Part model, mm, in its own coordinate system. A direction names the side the tool comes from. Round coordinates to 2 decimals unless told otherwise and drop trailing zeros. Order: outer loops, then holes, each group sorted by start corner. A loop starts at its lowest first (then second) coordinate and runs counter-clockwise, first axis right, second up. Notation, with made-up numbers: (30.5, 55) -> (78.5, 55) arc R21 cw to (78.5, 67) -> close; hole circle Ø11 at (6.25, -14). An arc over 180 degrees is marked (long way). Use CSV: the item, a comma, the result in double quotes.
```python
from build123d import *

# Parameters (mm, degrees)
SKETCH1_R              = 2.035533906
SKETCH1_R_2            = 1.5
BOSS_EXTRUDE1_DEPTH    = 1
SKETCH1_3_R            = 1.5
BOSS_EXTRUDE2_DEPTH    = 2
BOSS_EXTRUDE2_2_DEPTH  = 2
BOSS_EXTRUDE2_3_DEPTH  = 2
BOSS_EXTRUDE2_4_DEPTH  = 2
BOSS_EXTRUDE2_5_DEPTH  = 2
BOSS_EXTRUDE2_6_DEPTH  = 2
BOSS_EXTRUDE2_7_DEPTH  = 2
BOSS_EXTRUDE2_8_DEPTH  = 2
BOSS_EXTRUDE2_9_DEPTH  = 2
BOSS_EXTRUDE2_10_DEPTH = 2
BOSS_EXTRUDE2_11_DEPTH = 2
BOSS_EXTRUDE2_12_DEPTH = 2
BOSS_EXTRUDE2_13_DEPTH = 2
BOSS_EXTRUDE2_14_DEPTH = 2
BOSS_EXTRUDE2_15_DEPTH = 2
BOSS_EXTRUDE2_16_DEPTH = 2
SKETCH1_4_W            = 20
SKETCH1_4_H            = 20
BOSS_EXTRUDE3_DEPTH    = 1


with BuildPart() as part:
    # Sketch1 → Boss-Extrude1 (new body)
    with BuildSketch(Plane(origin=(0, 0, 0), x_dir=(1, 0, 0), z_dir=(0, 1, 0))):
        Polygon((1, 7.499999998), (1, 12.5), (1, 17.5), (0, 17.5), (0, 0), (20, 0), (20, 20), (2.5, 20), (2.5, 19), (7.5, 19), (12.500000017, 19), (17.5, 19), (19, 19), (19, 17.5), (19, 12.5), (19, 7.5), (19, 2.5), (19, 1), (17.5, 1), (12.49999999, 1), (7.5, 1), (2.5, 1), (1, 1), (1, 2.5), align=None)
        with Locations((5, 5)):
            Circle(SKETCH1_R)
        with Locations((5, 5)):
            Circle(SKETCH1_R_2, mode=Mode.SUBTRACT)
        with Locations((5, 10)):
            Circle(SKETCH1_R)
        with Locations((5, 10)):
            Circle(SKETCH1_R_2, mode=Mode.SUBTRACT)
        with BuildLine():
            ThreePointArc((3.560660176, 16.439339833), (2.964466094, 15.000000004), (3.560660171, 13.560660172))
            Line((3.560660172, 13.560660172), (3.939339828, 13.939339828))
            ThreePointArc((3.939339828, 13.939339828), (3.939339828, 16.060660172), (6.060660172, 16.060660172))
            Line((6.060660172, 16.060660172), (6.439339828, 16.439339828))
            ThreePointArc((6.439339828, 16.439339829), (5.000000003, 17.035533906), (3.560660176, 16.439339833))
        make_face()
        with BuildLine():
            Line((3.939339828, 13.939339828), (3.560660172, 13.560660172))
            ThreePointArc((3.560660171, 13.560660172), (5, 12.964466094), (6.439339828, 13.560660172))
            ThreePointArc((6.439339828, 13.560660172), (6.880588113, 14.221034898), (7.035533906, 15))
            ThreePointArc((7.035533906, 15), (6.880588113, 15.778965102), (6.439339828, 16.439339829))
            Line((6.439339828, 16.439339828), (6.060660172, 16.060660172))
            ThreePointArc((6.060660172, 16.060660172), (6.385819299, 15.574025149), (6.5, 15))
            ThreePointArc((6.5, 15), (5.574025149, 13.614180701), (3.939339828, 13.939339828))
        make_face()
        with Locations((10, 5)):
            Circle(SKETCH1_R)
        with Locations((10, 5)):
            Circle(SKETCH1_R_2, mode=Mode.SUBTRACT)
        with Locations((15, 5)):
            Circle(SKETCH1_R)
        with Locations((15, 5)):
            Circle(SKETCH1_R_2, mode=Mode.SUBTRACT)
        with Locations((15, 15)):
            Circle(SKETCH1_R)
        with Locations((15, 15)):
            Circle(SKETCH1_R_2, mode=Mode.SUBTRACT)
        with Locations((15, 10)):
            Circle(SKETCH1_R)
        with Locations((15, 10)):
            Circle(SKETCH1_R_2, mode=Mode.SUBTRACT)
        with Locations((10, 10)):
            Circle(SKETCH1_R)
        with Locations((10, 10)):
            Circle(SKETCH1_R_2, mode=Mode.SUBTRACT)
        with Locations((10, 15)):
            Circle(SKETCH1_R)
        with Locations((10, 15)):
            Circle(SKETCH1_R_2, mode=Mode.SUBTRACT)
        Polygon((0, 17.5), (1, 17.5), (1, 19), (2.5, 19), (2.5, 20), (0, 20), align=None)
    extrude(amount=-BOSS_EXTRUDE1_DEPTH)



with BuildPart() as body_2:
    # Sketch1_3 → Boss-Extrude2 (new body)
    with BuildSketch(Plane(origin=(0, 0, 0), x_dir=(1, 0, 0), z_dir=(0, 1, 0))):
        with Locations((2.5, 12.5)):
            Circle(SKETCH1_3_R)
    extrude(amount=BOSS_EXTRUDE2_DEPTH)


with BuildPart() as body_3:
    # Sketch1_3 → Boss-Extrude2 2 (new body)
    with BuildSketch(Plane(origin=(0, 0, 0), x_dir=(1, 0, 0), z_dir=(0, 1, 0))):
        with Locations((2.5, 17.5)):
            Circle(SKETCH1_3_R)
    extrude(amount=BOSS_EXTRUDE2_2_DEPTH)


with BuildPart() as body_4:
    # Sketch1_3 → Boss-Extrude2 3 (new body)
    with BuildSketch(Plane(origin=(0, 0, 0), x_dir=(1, 0, 0), z_dir=(0, 1, 0))):
        with Locations((7.5, 12.5)):
            Circle(SKETCH1_3_R)
    extrude(amount=BOSS_EXTRUDE2_3_DEPTH)


with BuildPart() as body_5:
    # Sketch1_3 → Boss-Extrude2 4 (new body)
    with BuildSketch(Plane(origin=(0, 0, 0), x_dir=(1, 0, 0), z_dir=(0, 1, 0))):
        with Locations((2.5, 7.5)):
            Circle(SKETCH1_3_R)
    extrude(amount=BOSS_EXTRUDE2_4_DEPTH)


with BuildPart() as body_6:
    # Sketch1_3 → Boss-Extrude2 5 (new body)
    with BuildSketch(Plane(origin=(0, 0, 0), x_dir=(1, 0, 0), z_dir=(0, 1, 0))):
        with Locations((7.5, 17.5)):
            Circle(SKETCH1_3_R)
    extrude(amount=BOSS_EXTRUDE2_5_DEPTH)


with BuildPart() as body_7:
    # Sketch1_3 → Boss-Extrude2 6 (new body)
    with BuildSketch(Plane(origin=(0, 0, 0), x_dir=(1, 0, 0), z_dir=(0, 1, 0))):
        with Locations((2.5, 2.5)):
            Circle(SKETCH1_3_R)
    extrude(amount=BOSS_EXTRUDE2_6_DEPTH)


with BuildPart() as body_8:
    # Sketch1_3 → Boss-Extrude2 7 (new body)
    with BuildSketch(Plane(origin=(0, 0, 0), x_dir=(1, 0, 0), z_dir=(0, 1, 0))):
        with Locations((12.5, 12.5)):
            Circle(SKETCH1_3_R)
    extrude(amount=BOSS_EXTRUDE2_7_DEPTH)


with BuildPart() as body_9:
    # Sketch1_3 → Boss-Extrude2 8 (new body)
    with BuildSketch(Plane(origin=(0, 0, 0), x_dir=(1, 0, 0), z_dir=(0, 1, 0))):
        with Locations((7.5, 7.5)):
            Circle(SKETCH1_3_R)
    extrude(amount=BOSS_EXTRUDE2_8_DEPTH)


with BuildPart() as body_10:
    # Sketch1_3 → Boss-Extrude2 9 (new body)
    with BuildSketch(Plane(origin=(0, 0, 0), x_dir=(1, 0, 0), z_dir=(0, 1, 0))):
        with Locations((12.5, 17.5)):
            Circle(SKETCH1_3_R)
    extrude(amount=BOSS_EXTRUDE2_9_DEPTH)


with BuildPart() as body_11:
    # Sketch1_3 → Boss-Extrude2 10 (new body)
    with BuildSketch(Plane(origin=(0, 0, 0), x_dir=(1, 0, 0), z_dir=(0, 1, 0))):
        with Locations((7.5, 2.5)):
            Circle(SKETCH1_3_R)
    extrude(amount=BOSS_EXTRUDE2_10_DEPTH)


with BuildPart() as body_12:
    # Sketch1_3 → Boss-Extrude2 11 (new body)
    with BuildSketch(Plane(origin=(0, 0, 0), x_dir=(1, 0, 0), z_dir=(0, 1, 0))):
        with Locations((17.5, 17.5)):
            Circle(SKETCH1_3_R)
    extrude(amount=BOSS_EXTRUDE2_11_DEPTH)


with BuildPart() as body_13:
    # Sketch1_3 → Boss-Extrude2 12 (new body)
    with BuildSketch(Plane(origin=(0, 0, 0), x_dir=(1, 0, 0), z_dir=(0, 1, 0))):
        with Locations((17.5, 12.5)):
            Circle(SKETCH1_3_R)
    extrude(amount=BOSS_EXTRUDE2_12_DEPTH)


with BuildPart() as body_14:
    # Sketch1_3 → Boss-Extrude2 13 (new body)
    with BuildSketch(Plane(origin=(0, 0, 0), x_dir=(1, 0, 0), z_dir=(0, 1, 0))):
        with Locations((12.5, 7.5)):
            Circle(SKETCH1_3_R)
    extrude(amount=BOSS_EXTRUDE2_13_DEPTH)


with BuildPart() as body_15:
    # Sketch1_3 → Boss-Extrude2 14 (new body)
    with BuildSketch(Plane(origin=(0, 0, 0), x_dir=(1, 0, 0), z_dir=(0, 1, 0))):
        with Locations((12.5, 2.5)):
            Circle(SKETCH1_3_R)
    extrude(amount=BOSS_EXTRUDE2_14_DEPTH)


with BuildPart() as body_16:
    # Sketch1_3 → Boss-Extrude2 15 (new body)
    with BuildSketch(Plane(origin=(0, 0, 0), x_dir=(1, 0, 0), z_dir=(0, 1, 0))):
        with Locations((17.5, 2.5)):
            Circle(SKETCH1_3_R)
    extrude(amount=BOSS_EXTRUDE2_15_DEPTH)


with BuildPart() as body_17:
    # Sketch1_3 → Boss-Extrude2 16 (new body)
    with BuildSketch(Plane(origin=(0, 0, 0), x_dir=(1, 0, 0), z_dir=(0, 1, 0))):
        with Locations((17.5, 7.5)):
            Circle(SKETCH1_3_R)
    extrude(amount=BOSS_EXTRUDE2_16_DEPTH)


with BuildPart() as part_1:
    add(part.part)

    add(body_2.part)  # Boss-Extrude3 merges body 2

    add(body_3.part)  # Boss-Extrude3 merges body 3

    add(body_4.part)  # Boss-Extrude3 merges body 4

    add(body_5.part)  # Boss-Extrude3 merges body 5

    add(body_6.part)  # Boss-Extrude3 merges body 6

    add(body_7.part)  # Boss-Extrude3 merges body 7

    add(body_8.part)  # Boss-Extrude3 merges body 8

    add(body_9.part)  # Boss-Extrude3 merges body 9

    add(body_10.part)  # Boss-Extrude3 merges body 10

    add(body_11.part)  # Boss-Extrude3 merges body 11

    add(body_12.part)  # Boss-Extrude3 merges body 12

    add(body_13.part)  # Boss-Extrude3 merges body 13

    add(body_14.part)  # Boss-Extrude3 merges body 14

    add(body_15.part)  # Boss-Extrude3 merges body 15

    add(body_16.part)  # Boss-Extrude3 merges body 16

    add(body_17.part)  # Boss-Extrude3 merges body 17
    # Sketch1_4 → Boss-Extrude3 (add)
    with BuildSketch(Plane(origin=(0, 0, 0), x_dir=(1, 0, 0), z_dir=(0, 1, 0))):
        with Locations((10, 10)):
            Rectangle(SKETCH1_4_W, SKETCH1_4_H)
    extrude(amount=BOSS_EXTRUDE3_DEPTH)


solid = part_1.part
```
(1) Cut at D-D, the plane z = -7.5. Give the cut face in (x, y).
Reply:
outline,"(0, -1) -> (1, -1) -> (1, 0) -> (19, 0) -> (19, -1) -> (20, -1) -> (20, 1) -> (19, 1) -> (19, 2) -> (16, 2) -> (16, 1) -> (14, 1) -> (14, 2) -> (11, 2) -> (11, 1) -> (9, 1) -> (9, 2) -> (6, 2) -> (6, 1) -> (4, 1) -> (4, 2) -> (1, 2) -> (1, 1) -> (0, 1) -> close"
(2) Pull direction Z, two halves, no side cores. Call faces 3 (the face through (5, 0, -15)), 4 (the face through (0, 0, -10)), 5 (the face through (10, 0, 0)): released by +Z, released by -Z, zero draft, split by the parting line, or undercut.
Reply:
face 3,"undercut"
face 4,"zero draft"
face 5,"released by +Z"
(3) Probe probe 1 along X at (y, z) = (-0.45, -2.5); probe 2 along Y at (x, z) = (12.75, -7.75); probe 3 along Y at (x, z) = (3.75, -10.25). List the from-to ranges inside material, lowest first. Write a range as [from, to].
Reply:
probe 1,"[0, 1], [19, 20]"
probe 2,"[0, 2]"
probe 3,"[0, 1]"
(4) Drop flat-ended pins along their axis: P1, Ø2.5, axis at x = 10, z = -15, coming from the -Y side; P2, Ø1.8, axis at x = 5, z = -10, coming from the +Y side. Give the stop position or say it passes through.
Reply:
P1,"y = 0"
P2,"y = 1"
(5) Cut at B-B, the plane y = 1.7. State how many separate pieces and enclosed holes the cut face has, then the cut area to 3 significant figures.
Reply:
separate pieces,"16"
enclosed holes,"0"
area,"113 mm2"
(6) Which spindle directions (+Z, -Z, +X, -X, +Y, -Y) get a long thin tool onto all of the face, cutting with end or side? Do faces 1 (the face through (17, 2, -8)), 2 (the face through (13.5, -0.49, -15.07)). Say none if no direction does.
Reply:
face 1,"+Z, -Z, +X, -X, +Y"
face 2,"-Y"
